```python
from build123d import *

# Parameters (mm, degrees)
SKETCH_W        = 50.8
SKETCH_H        = 25.4
SKETCH_R        = 1.27
SKETCH_W_2      = 6.35
SKETCH_H_2      = 0.762
PAD_DEPTH       = 1.905
SKETCH001_W     = 50.8
SKETCH001_H     = 25.4
PAD001_DEPTH    = 7.62
SKETCH002_R     = 3.302
SKETCH002_R_2   = 4.445
POCKET_DEPTH    = 7.62
SKETCH003_W     = 50.8
SKETCH003_H     = 6.35
PAD002_DEPTH    = 2.54
SKETCH004_W     = 8.89
SKETCH004_H     = 3.81
PAD003_DEPTH    = 6.35
SKETCH005_R     = 1.7653
POCKET001_DEPTH = 5.08
FILLET_R        = 5.08
FILLET001_R     = 2.032
FILLET002_R     = 3.81
CHAMFER_SIZE    = 2.286


with BuildPart() as part:
    # Sketch → Pad (new body)
    with BuildSketch(Plane.XY):
        Rectangle(SKETCH_W, SKETCH_H)
        with Locations((-19.05, 0)):
            Circle(SKETCH_R, mode=Mode.SUBTRACT)
        with Locations((19.05, 0)):
            Circle(SKETCH_R, mode=Mode.SUBTRACT)
        with Locations((6.985, -4.826)):
            Rectangle(SKETCH_W_2, SKETCH_H_2, mode=Mode.SUBTRACT)
        with Locations((-6.985, -4.826)):
            Rectangle(SKETCH_W_2, SKETCH_H_2, mode=Mode.SUBTRACT)
    extrude(amount=PAD_DEPTH)

    # Sketch001 (on Face16 of Pad) → Pad001 (join)
    with BuildSketch(Plane.XY.offset(1.905)):
        Rectangle(SKETCH001_W, SKETCH001_H)
    extrude(amount=PAD001_DEPTH)

    # Sketch002 (on Face17 of Pad001) → Pocket (cut)
    with BuildSketch(Plane.XY.offset(9.525)):
        with Locations((-6.985, -4.445)):
            Circle(SKETCH002_R)
        with Locations((6.985, -4.445)):
            Circle(SKETCH002_R)
        with Locations((19.05, 0)):
            Circle(SKETCH002_R_2)
        with Locations((-19.05, 0)):
            Circle(SKETCH002_R_2)
    extrude(amount=-POCKET_DEPTH, mode=Mode.SUBTRACT)

    # Sketch003 (on Face1 of Pocket) → Pad002 (join)
    with BuildSketch(Plane(origin=(0, 0, 0), x_dir=(1, 0, 0), z_dir=(0, 0, -1))):
        with Locations((0, -9.525)):
            Rectangle(SKETCH003_W, SKETCH003_H)
    extrude(amount=PAD002_DEPTH)

    # Sketch004 (on Face15 of Pad002) → Pad003 (join)
    with BuildSketch(Plane.XY.offset(9.525)):
        with Locations((0, 10.795)):
            Rectangle(SKETCH004_W, SKETCH004_H)
    extrude(amount=PAD003_DEPTH)

    # Sketch005 (on Face23 of Pad003) → Pocket001 (cut)
    with BuildSketch(Plane.XZ.offset(-8.89)):
        with Locations((0, 12.7)):
            Circle(SKETCH005_R)
    extrude(amount=-POCKET001_DEPTH, mode=Mode.SUBTRACT)

    # Fillet
    fillet_edges = [part.edges().sort_by_distance(p)[0] for p in [
        (25.4, 12.7, 3.4925),
        (-25.4, 12.7, 3.4925),
        (25.4, -12.7, 4.7625),
        (-25.4, -12.7, 4.7625),
    ]]
    fillet(fillet_edges, radius=FILLET_R)

    # Fillet001
    fillet001_edges = [part.edges().sort_by_distance(p)[0] for p in [
        (4.445, 10.795, 9.525),
        (-4.445, 10.795, 9.525),
    ]]
    fillet(fillet001_edges, radius=FILLET001_R)

    # Fillet002
    fillet002_edges = [part.edges().sort_by_distance(p)[0] for p in [
        (-4.445, 10.795, 15.875),
        (4.445, 10.795, 15.875),
    ]]
    fillet(fillet002_edges, radius=FILLET002_R)

    # Chamfer
    chamfer_edges = [part.edges().sort_by_distance(p)[0] for p in [
        (0, 6.35, -2.54),
    ]]
    chamfer(chamfer_edges, length=CHAMFER_SIZE)


solid = part.part
```
CAD build for the part. Positions are in the model's coordinates, mm. A direction names the side the tool comes from. Give positions to 0.01 mm unless a question says otherwise; leave off trailing zeros. Loops run counter-clockwise (first coordinate to the right, second up) from the corner with the lowest first, then second, coordinate; pieces in that order, holes last. Notation, with made-up numbers: M 33.5,14 L 74.5,14 A22 ccw 74.5,40 Z; hole C 65,7.5 d6. An arc over 180 degrees is marked long. Use one line per item in the form item = value.
Item 1: Flat gauge pins, fed straight in: pin 1 (8 mm diameter, centred on x = 19.05, y = 0, fed in from +Z) (3 decimals); pin 2 (8 mm diameter, centred on x = -11.5, y = 1, fed in from -Z); pin 3 (5 mm diameter, centred on x = 17.5, y = -4, fed in from +Z) (3 decimals). Where does each tip first touch, or does it go through?
Determined:
pin_1 = 1.905
pin_2 = 0
pin_3 = 9.525
Item 2: Slice it at D-D (z = 12.7). List the corners of the cut face in (x, y), plus the area to 3 significant figures.
Determined:
outline = M -4.39,8.89 L -1.77,8.89 L -1.77,12.7 L -4.39,12.7 Z; M 1.77,8.89 L 4.39,8.89 L 4.39,12.7 L 1.77,12.7 Z
area = 20.0 mm2
Item 3: Slice it at A-A (y = 0). List the corners of the cut face in (x, z) (3 decimals), plus the area to 3 significant figures.
Determined:
outline = M -25.4,0 L -20.32,0 L -20.32,1.905 L -23.495,1.905 L -23.495,9.525 L -25.4,9.525 Z; M -17.78,0 L 17.78,0 L 17.78,1.905 L 14.605,1.905 L 14.605,9.525 L -14.605,9.525 L -14.605,1.905 L -17.78,1.905 Z; M 20.32,0 L 25.4,0 L 25.4,9.525 L 23.495,9.525 L 23.495,1.905 L 20.32,1.905 Z
area = 339 mm2
Item 4: Drill centre lines: probe 1 along Y at (x, z) = (19.05, 4.5) (3 decimals); probe 2 along Z at (x, y) = (-22, -8.75) (3 decimals); probe 3 along Y at (x, z) = (-20.5, 1.75). Where is each one in solid material? Low to high. Write a range as from..to.
Determined:
probe_1 = -12.7..-4.445, 4.445..12.7
probe_2 = 0..9.525
probe_3 = -12.7..12.7
Item 5: Two-plate mould, pull along Y, no slides. Class faces 4 (the face through (-23.951, 11.172, 3.408)), 5 (the face through (-23.951, -11.172, 4.829)), 6 (the face through (3.3, 10.82, 14.79)), 7 (the face through (23.3, 1.3, 5.8)): pulls with the +Y half, pulls with the -Y half, needs draft (parallel to the pull), parting line crosses it, or undercut.
Determined:
face_4 = pulls with the +Y half
face_5 = pulls with the -Y half
face_6 = needs draft
face_7 = undercut
Item 6: Slice it at B-B (x = 0). List the corners of the cut face in (y, z) (3 decimals).
Determined:
outline = M -12.7,0 L 6.35,0 L 6.35,-0.254 L 8.636,-2.54 L 12.7,-2.54 L 12.7,10.935 L 8.89,10.935 L 8.89,9.525 L -12.7,9.525 Z; M 8.89,14.465 L 12.7,14.465 L 12.7,15.875 L 8.89,15.875 Z
Item 7: Slice it at C-C (z = 7). List the corners of the cut face in (x, y) (3 decimals).
Determined:
outline = M -25.4,-7.62 A5.08 ccw -20.32,-12.7 L 20.32,-12.7 A5.08 ccw 25.4,-7.62 L 25.4,7.62 A5.08 ccw 20.32,12.7 L -20.32,12.7 A5.08 ccw -25.4,7.62 Z; hole C -19.05,0 d8.89; hole C -6.985,-4.445 d6.604; hole C 6.985,-4.445 d6.604; hole C 19.05,0 d8.89
Item 8: Which spindle directions (+Z, -Z, +X, -X, +Y, -Y) get a long thin tool onto all of the face, cutting with end or side? Do faces 1 (the face through (17.78, 0.06, 0.94)), 2 (the face through (0, -3, 0)), 3 (the face through (7, -4, 1.905)). Say none if no direction does.
Determined:
face_1 = +Z, -Z
face_2 = -Z, +X, -X, -Y
face_3 = +Z
